The model under review builds one solid part; all positions refer to its coordinate system, in mm. Round coordinates to 2 decimals unless told otherwise and drop trailing zeros. Write each loop counter-clockwise with the first axis right and the second up, starting at its lowest first coordinate (ties: lowest second). Pieces come first, ordered by that corner, then holes. Notation, with made-up numbers: (81.25, 60.5) -> (107.25, 60.5) arc R9 ccw to (107.25, 73.5) -> close; hole circle Ø7 at (49.5, 12.25). An arc over 180 degrees is marked (long way). Answer as a JSON object with one key per item and string values. Group by question number.
1) We need section A-A, the plane y = 0. Write out the cut boundary in (x, z), then the cut area to 3 significant figures.
2) To check wall thickness, follow probe 1 along X at (y, z) = (-0.5, 0.55); probe 2 along X at (y, z) = (-1, 0.2); probe 3 along Y at (x, z) = (10, 0.8). State the ranges of each line that lie inside material, in increasing order. Write a range as [from, to].
3) We need section B-B, the plane z = 0.6. Write out the cut boundary in (x, y) (3 decimals), then the cut area to 3 significant figures.
4) We need section D-D, the plane y = 1. Write out the cut boundary in (x, z).
5) Mouldability with a two-part tool opening along X and no side actions: class faces 1 (the flat face through (0, 0, 1)), 2 (the cylindrical face through (-8.75, -0.05, 0.49)), 3 (the cylindrical face through (-13, -0.1, 0.5)) as pulls with the +X half, pulls with the -X half, needs draft (parallel to the pull), parting line crosses it, or undercut.
6) We need section C-C, the plane x = 10. Write out the cut boundary in (y, z).
from build123d import *

# Parameters (mm, degrees)
CROQUIS1_R              = 1.25
SALIENTE_EXTRUIR1_DEPTH = 1


with BuildPart() as part:
    # Croquis1 → Saliente-Extruir1 (new body)
    with BuildSketch(Plane.XY):
        with BuildLine():
            Line((3, 3.875), (10.362810685, 2.977980592))
            ThreePointArc((10.362810685, 2.977980592), (13, 0), (10.362810685, -2.977980592))
            Line((10.362810685, -2.977980592), (3, -3.875))
            Line((3, -3.875), (-3, -3.875))
            Line((-3, -3.875), (-10.362810685, -2.977980592))
            ThreePointArc((-10.362810685, -2.977980592), (-13, 0), (-10.362810685, 2.977980592))
            Line((-10.362810685, 2.977980592), (-3, 3.875))
            Line((-3, 3.875), (3, 3.875))
        make_face()
        with Locations((10, 0)):
            Circle(CROQUIS1_R, mode=Mode.SUBTRACT)
        with Locations(Location((-10, 0, 0), (0, 0, 180))):
            Circle(CROQUIS1_R, mode=Mode.SUBTRACT)
    extrude(amount=SALIENTE_EXTRUIR1_DEPTH)


solid = part.part
Here are the results:
{
 "1": {"outline": "(-13, 0) -> (-11.25, 0) -> (-11.25, 1) -> (-13, 1) -> close; (-8.75, 0) -> (8.75, 0) -> (8.75, 1) -> (-8.75, 1) -> close; (11.25, 0) -> (13, 0) -> (13, 1) -> (11.25, 1) -> close", "area": "21.0 mm^2"},
 "2": {"probe 1": "x = [-12.96, -11.15], [-8.85, 8.85], [11.15, 12.96]", "probe 2": "x = [-12.83, -10.75], [-9.25, 9.25], [10.75, 12.83]", "probe 3": "y = [-3.02, -1.25], [1.25, 3.02]"},
 "3": {"outline": "(-10.363, -2.978) -> (-3, -3.875) -> (3, -3.875) -> (10.363, -2.978) arc R3 ccw to (10.363, 2.978) -> (3, 3.875) -> (-3, 3.875) -> (-10.363, 2.978) arc R3 ccw to start; hole circle Ø2.5 at (-10, 0); hole circle Ø2.5 at (10, 0)", "area": "162 mm^2"},
 "4": {"outline": "(-12.83, 0) -> (-10.75, 0) -> (-10.75, 1) -> (-12.83, 1) -> close; (-9.25, 0) -> (9.25, 0) -> (9.25, 1) -> (-9.25, 1) -> close; (10.75, 0) -> (12.83, 0) -> (12.83, 1) -> (10.75, 1) -> close"},
 "5": {"face 1": "needs draft", "face 2": "undercut", "face 3": "pulls with the -X half"},
 "6": {"outline": "(-3.02, 0) -> (-1.25, 0) -> (-1.25, 1) -> (-3.02, 1) -> close; (1.25, 0) -> (3.02, 0) -> (3.02, 1) -> (1.25, 1) -> close"}
}
